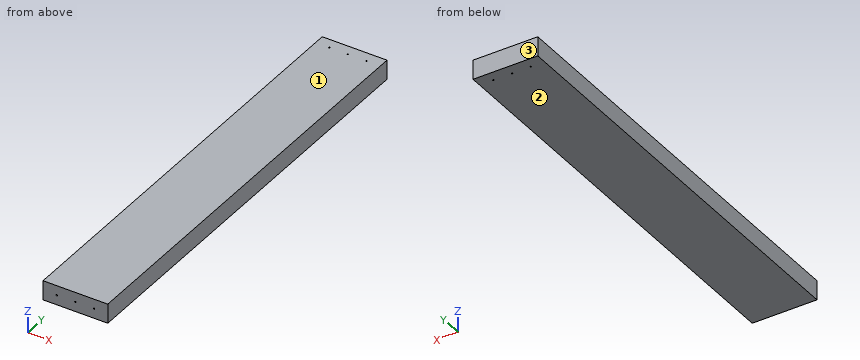
from build123d import *

# Parameters (mm, degrees)
SKETCH2_W               = 63.5
SKETCH2_H               = 19.05
BOSS_EXTRUDE1_DEPTH     = 425.45
CUT_EXTRUDE1_DEPTH      = 431.584318107
CUT_EXTRUDE1_DEPTH_BACK = 50.8
SKETCH3_R               = 0.635
SKETCH4_R               = 0.635
CUT_EXTRUDE2_DEPTH      = 431.584318107


with BuildPart() as part:
    # Sketch2 → Boss-Extrude1 (new body)
    with BuildSketch(Plane(origin=(0, 0, 0), x_dir=(1, 0, 0), z_dir=(0, 1, 0))):
        with Locations((31.75, 9.525)):
            Rectangle(SKETCH2_W, SKETCH2_H)
    extrude(amount=BOSS_EXTRUDE1_DEPTH)

    # Sketch3 → Cut-Extrude1 (cut, two sides: drawn at the far end of the back side and taken through both)
    with BuildSketch(Plane.XZ.offset(-CUT_EXTRUDE1_DEPTH_BACK)):
        with Locations(Location((13.4874, -9.525, 0), (0, 0, 270))):
            Circle(SKETCH3_R)
        with Locations(Location((31.75, -9.525, 0), (0, 0, 270))):
            Circle(SKETCH3_R)
        with Locations(Location((50.0126, -9.525, 0), (0, 0, 270))):
            Circle(SKETCH3_R)
    extrude(amount=CUT_EXTRUDE1_DEPTH + CUT_EXTRUDE1_DEPTH_BACK, mode=Mode.SUBTRACT)

    # Sketch4 → Cut-Extrude2 (cut, through all)
    with BuildSketch(Plane.XY):
        with Locations((31.75, 415.29)):
            Circle(SKETCH4_R)
        with Locations((50.0126, 415.29)):
            Circle(SKETCH4_R)
        with Locations(Location((13.4874, 415.29, 0), (0, 0, 180))):
            Circle(SKETCH4_R)
    extrude(amount=-CUT_EXTRUDE2_DEPTH, mode=Mode.SUBTRACT)


solid = part.part
Could you check a few things on this model? Use its own coordinates, in mm. Face numbers are marked on the shaded views. Coordinates: 2 decimals unless noted, no trailing zeros. One line per item, written item: value. Start each with the question number.
1) If I drill on L1, parallel to X at y = 415.29, z = -9.5 (3 decimals); L2, parallel to Z at x = 32, y = 31; L3, parallel to Y at x = 13.5, z = -10, over which ranges is the centre line in solid material (lowest first)? Write a range as [from, to].
2) I'm going to push flat-ended pins straight in: pin 1 (1 mm diameter, centred on x = 31.75, y = 415.29, fed in from -Z); pin 2 (0.8 mm diameter, centred on x = 50.01, z = -9.52, fed in from -Y). Where does each tip first touch, or does it pass through?
3) We'd pull the mould along Z, two halves only. Please class the marked faces 1, 2 and 3: +Z half, -Z half, draft (parallel to the pull), parting line (faces both ways), or undercut.
Answer list:
1. L1: x = [0, 12.852], [14.122, 31.115], [32.385, 49.378], [50.648, 63.5]
1. L2: z = [-19.05, -10.11], [-8.94, 0]
1. L3: y = [50.8, 414.66], [415.92, 425.45]
2. pin 1: passes through
2. pin 2: stops at y = 50.8
3. face 1: +Z half
3. face 2: -Z half
3. face 3: draft
